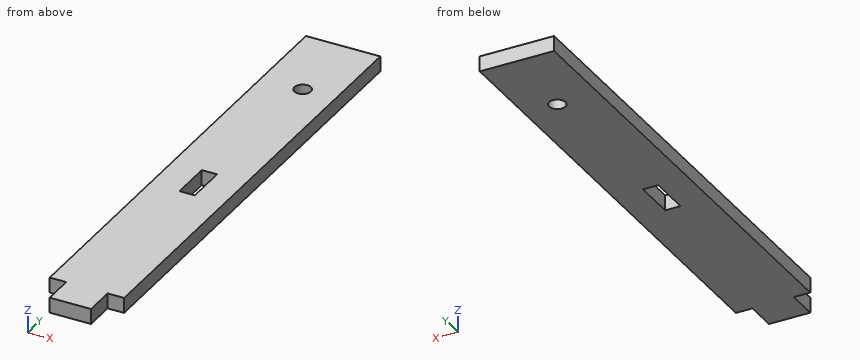
Autodesk Inventor part; units mm, degrees
ref_plane "YZ Plane" through (0, 0, 0) normal (1, 0, 0) x (0, 1, 0)
ref_plane "XZ Plane" through (0, 0, 0) normal (0, 1, 0) x (-1, 0, 0)
ref_plane "XY Plane" through (0, 0, 0) normal (0, 0, 1) x (1, 0, 0)
sketch "Sketch1" plane through (0, 0, 0) normal (0, 0, 1) x (1, 0, 0)
  line L0 (0, 0) -> (0, 575)
  line L1 (0, 575) -> (90, 575)
  line L2 (90, 575) -> (90, 0)
  line L3 (90, 0) -> (0, 0)
  dimension "d0" = 575
  dimension "d1" = 90
extrude "Extrusion1" add sketch "Sketch1" along normal blind 18.55
sketch "Sketch2" plane through (0, 0, 18.55) normal (0, 0, 1) x (1, 0, 0)
  circle A0 centre (50, 475) radius 10
  line L0 (0, 575) -> (0, 0)
  line L1 (0, 475) -> (90, 475) construction
  line L2 (90, 0) -> (90, 575)
  line L3 (90, 575) -> (0, 575)
  dimension "d4" = 50
  dimension "d5" = 100
  dimension "d6" = 20
extrude "Extrusion2" cut sketch "Sketch2" against normal blind 100
sketch "Sketch3" plane through (0, 0, 18.55) normal (0, 0, 1) x (1, 0, 0)
  line L0 (0, 0) -> (90, 0)
  line L1 (20, 0) -> (70, 0)
  line L2 (70, 0) -> (70, -37.1)
  line L3 (70, -37.1) -> (20, -37.1)
  line L4 (20, -37.1) -> (20, 0)
  line L5 (0, 575) -> (0, 0)
  line L6 (90, 0) -> (90, 575)
  dimension "d9" = 20
  dimension "d10" = 20
  dimension "d11" = 37.1
extrude "Extrusion3" add sketch "Sketch3" against normal blind 18.55
sketch "Sketch4" plane through (0, 0, 18.55) normal (0, 0, 1) x (1, 0, 0)
  line L0 (35.7, 275) -> (54.3, 275)
  line L1 (54.3, 275) -> (54.3, 225)
  line L2 (54.3, 225) -> (35.7, 225)
  line L3 (35.7, 225) -> (35.7, 275)
  line L4 (90, 575) -> (0, 575)
  line L5 (35.7, 250) -> (0, 250) construction
  line L6 (0, 575) -> (0, 0)
  line L7 (54.3, 250) -> (90, 250) construction
  line L8 (90, 0) -> (90, 575)
  dimension "d14" = 300
  dimension "d15" = 50
  dimension "d16" = 18.6
extrude "Extrusion4" cut sketch "Sketch4" against normal blind 200
properties part number "table_foot"
The listing builds one solid part. Answer for the finished solid, in the listing's coordinates (mm). Round coordinates to 2 decimals unless told otherwise and drop trailing zeros. Write each loop counter-clockwise with the first axis right and the second up, starting at its lowest first coordinate (ties: lowest second). Pieces come first, ordered by that corner, then holes. Notation, with made-up numbers: (-20, 49.5) -> (0, 49.5) arc R7 ccw to (0, 60.5) -> close; hole circle Ø2 at (51.5, 24). An arc over 180 degrees is marked (long way). Use CSV: the item, a comma, the result in double quotes. Start each with the question number.
(1) Consider L1, parallel to Y at x = 50, z = 4.5; L2, parallel to Y at x = 38, z = 13.5; L3, parallel to Y at x = 71.5, z = 2.75. Determine where each line is inside the solid, lowest interval first. Write a range as from..to.
(2) Section A-A on y = 475 is taken. Give the vertices of the cut face in (x, z), then the cut area to 3 significant figures.
(3) Section D-D on x = 82 is taken. Give the vertices of the cut face in (y, z).
(4) Section B-B on z = 6.5 is taken. Give the vertices of the cut face in (x, y), then the cut area to 3 significant figures.
(5) Section C-C on y = 239 is taken. Give the vertices of the cut face in (x, z).
(6) Each of these flat-tipped pins is pushed along its axis until it touches: pin 1 (5.5 mm diameter, centred on y = -17, z = 9.5, fed in from -X); pin 2 (5.5 mm diameter, centred on y = -25, z = 11.5, fed in from +X). Where does it stop, or does it pass through?
A:
1,L1,"y = -37.1..225, 275..465, 485..575"
1,L2,"y = -37.1..225, 275..575"
1,L3,"y = 0..575"
2,outline,"(0, 0) -> (40, 0) -> (40, 18.55) -> (0, 18.55) -> close; (60, 0) -> (90, 0) -> (90, 18.55) -> (60, 18.55) -> close"
2,area,"1,300 mm²"
3,outline,"(0, 0) -> (575, 0) -> (575, 18.55) -> (0, 18.55) -> close"
4,outline,"(0, 0) -> (20, 0) -> (20, -37.1) -> (70, -37.1) -> (70, 0) -> (90, 0) -> (90, 575) -> (0, 575) -> close; hole (35.7, 225) -> (54.3, 225) -> (54.3, 275) -> (35.7, 275) -> close; hole circle Ø20 at (50, 475)"
4,area,"52,400 mm²"
5,outline,"(0, 0) -> (35.7, 0) -> (35.7, 18.55) -> (0, 18.55) -> close; (54.3, 0) -> (90, 0) -> (90, 18.55) -> (54.3, 18.55) -> close"
6,pin 1,"stops at x = 20"
6,pin 2,"stops at x = 70"
